Here's how the part is built. I have some questions about the finished solid (model axes, mm). A direction names the side the tool comes from. Coordinates: 2 decimals unless noted, no trailing zeros. Write each loop counter-clockwise with the first axis right and the second up, starting at its lowest first coordinate (ties: lowest second). Pieces come first, ordered by that corner, then holes.
Item 1: If we mould it in two halves opening along X, with no side actions, what happens to faces 1 (the face through (2, 70, 1)), 2 (the face through (-0.2, -44, 2)), 3 (the face through (0, 68, 1)), 4 (the face through (-15, -51, 1))? For each: pulls with the +X half, pulls with the -X half, needs draft (parallel to the pull), parting line crosses it, or undercut.
Item 2: I want a section at C-C (z = 1.75). Count the separate pieces of the cut face and the enclosed holes in it, and give its area (3 significant figures).
Item 3: I'm going to push flat-ended pins straight in: P1, Ø12, axis at x = -1.5, y = -0.5, coming from the -Z side; P2, Ø1.5, axis at y = -43, z = 1, coming from the +X side; P3, Ø1, axis at y = 17, z = 1.5, coming from the +X side; P4, Ø0.9, axis at x = -3.5, z = 1.5, coming from the +Y side. Where does each tip first touch, or does it pass through?
Item 4: Please list where these lines run through material, in increasing order: line 1 (Y direction, x = -1.5, z = 1.25); line 2 (Y direction, x = -10.25, z = 2.85); line 3 (X direction, y = 55.5, z = 1.5).
Item 5: I want a section at A-A (x = -8.75). Please give me the cut outline in (y, z), and give its area (3 significant figures).
Item 6: For faces 5 (the face through (-10, -50, 1)), 6 (the face through (-0.2, 61, 2)), 7 (the face through (-10, 69, 1)), 8 (the face through (-12, -52, 1)), which set-ups out of +Z, -Z, +X, -X, +Y, -Y let a thin tool reach every point of the face, with its end or its side?
Item 7: I want a section at B-B (x = -4). Please give me the cut outline in (y, z), and give its area (3 significant figures).
from build123d import *

# Parameters (mm, degrees)
CROQUIS1_W              = 10
CROQUIS1_H              = 3
SALIENTE_EXTRUIR1_DEPTH = 3
CROQUIS2_W              = 0.3
CROQUIS2_H              = 0.3
CROQUIS2_H_2            = 3
CORTAR_EXTRUIR2_DEPTH   = 3


with BuildPart() as part:
    # Croquis1 → Saliente-Extruir1 (new body)
    with BuildSketch(Plane.XY):
        with BuildLine():
            Line((-10, 70), (-10, 67))
            Line((-10, 67), (-7, 67))
            Line((-7, 67), (-7, 63))
            Line((-7, 63), (-9.5, 63))
            Line((-9.5, 63), (-9.5, 60))
            Line((-9.5, 60), (-0.5, 60))
            Line((-0.5, 60), (-0.5, 63))
            Line((-0.5, 63), (-3, 63))
            Line((-3, 63), (-3, 67))
            Line((-3, 67), (0, 67))
            Line((0, 67), (0, 70))
            Line((0, 70), (5, 70))
            Line((5, 70), (5, 67.405747627))
            ThreePointArc((5, 67.405747627), (4.929306729, 67.036438809), (4.727221995, 66.719345288))
            add(Edge.make_bspline(
                [(4.727221995, 66.719345288), (3.242407332, 65.146230192), (1.757592668, 62), (3.242407332, 58.853769808), (4.727221995, 57.280654712)],
                knots=[0.028065471, 0.028065471, 0.028065471, 0.028065471, 0.5, 0.971934529, 0.971934529, 0.971934529, 0.971934529], degree=3))
            ThreePointArc((4.727221995, 57.280654712), (4.929306729, 56.963561191), (5, 56.594252373))
            Line((5, 56.594252373), (5, 54.181314171))
            ThreePointArc((5, 54.181314171), (4.9841425, 54.003934523), (4.937072921, 53.832180471))
            add(Edge.make_bspline(
                [(4.937072921, 53.832180471), (3.31235764, 49.471453647), (1.68764236, 40.75), (3.31235764, 32.028546353), (4.937072921, 27.667819529)],
                knots=[0.006332812, 0.006332812, 0.006332812, 0.006332812, 0.5, 0.993667188, 0.993667188, 0.993667188, 0.993667188], degree=3))
            ThreePointArc((4.937072921, 27.667819529), (4.9841425, 27.496065477), (5, 27.318685829))
            Line((5, 27.318685829), (5, 24.567654138))
            ThreePointArc((5, 24.567654138), (4.997723384, 24.500214919), (4.990903903, 24.433082766))
            add(Edge.make_bspline(
                [(4.990903903, -48.933082766), (3.330301301, -36.70538851), (1.669698699, -12.25), (3.330301301, 12.20538851), (4.990903903, 24.433082766)],
                knots=[0.000910439, 0.000910439, 0.000910439, 0.000910439, 0.5, 0.999089561, 0.999089561, 0.999089561, 0.999089561], degree=3))
            ThreePointArc((4.990903903, -48.933082766), (4.997723384, -49.000214919), (5, -49.067654138))
            Line((5, -49.067654138), (5, -51.701381229))
            Line((5, -51.701381229), (5, -52))
            Line((5, -52), (0, -52))
            Line((0, -52), (0, -49))
            Line((0, -49), (-3, -49))
            Line((-3, -49), (-3, -45.5))
            Line((-3, -45.5), (-0.5, -45.5))
            Line((-0.5, -45.5), (-0.5, -42.5))
            Line((-0.5, -42.5), (-9.5, -42.5))
            Line((-9.5, -42.5), (-9.5, -45.5))
            Line((-9.5, -45.5), (-7, -45.5))
            Line((-7, -45.5), (-7, -49))
            Line((-7, -49), (-10, -49))
            Line((-10, -49), (-10, -52))
            Line((-10, -52), (-15, -52))
            Line((-15, -52), (-15, -51.701381229))
            Line((-15, -51.701381229), (-15, -49.067654138))
            ThreePointArc((-15, -49.067654138), (-14.997723384, -49.000214919), (-14.990903903, -48.933082766))
            add(Edge.make_bspline(
                [(-14.990903903, -48.933082766), (-13.330301301, -36.70538851), (-11.669698699, -12.25), (-13.330301301, 12.20538851), (-14.990903903, 24.433082766)],
                knots=[0.000910439, 0.000910439, 0.000910439, 0.000910439, 0.5, 0.999089561, 0.999089561, 0.999089561, 0.999089561], degree=3))
            ThreePointArc((-14.990903903, 24.433082766), (-14.997723384, 24.500214919), (-15, 24.567654138))
            Line((-15, 24.567654138), (-15, 27.318685829))
            ThreePointArc((-15, 27.318685829), (-14.9841425, 27.496065477), (-14.937072921, 27.667819529))
            add(Edge.make_bspline(
                [(-14.937072921, 53.832180471), (-13.31235764, 49.471453647), (-11.68764236, 40.75), (-13.31235764, 32.028546353), (-14.937072921, 27.667819529)],
                knots=[0.006332812, 0.006332812, 0.006332812, 0.006332812, 0.5, 0.993667188, 0.993667188, 0.993667188, 0.993667188], degree=3))
            ThreePointArc((-14.937072921, 53.832180471), (-14.9841425, 54.003934523), (-15, 54.181314171))
            Line((-15, 54.181314171), (-15, 56.594252373))
            ThreePointArc((-15, 56.594252373), (-14.929306729, 56.963561191), (-14.727221995, 57.280654712))
            add(Edge.make_bspline(
                [(-14.727221995, 57.280654712), (-13.242407332, 58.853769808), (-11.757592668, 62), (-13.242407332, 65.146230192), (-14.727221995, 66.719345288)],
                knots=[0.028065471, 0.028065471, 0.028065471, 0.028065471, 0.5, 0.971934529, 0.971934529, 0.971934529, 0.971934529], degree=3))
            ThreePointArc((-14.727221995, 66.719345288), (-14.929306729, 67.036438809), (-15, 67.405747627))
            Line((-15, 67.405747627), (-15, 70))
            Line((-15, 70), (-10, 70))
        make_face()
        with Locations((-5, 26)):
            Rectangle(CROQUIS1_W, CROQUIS1_H, mode=Mode.SUBTRACT)
        with Locations((-5, 55.5)):
            Rectangle(CROQUIS1_W, CROQUIS1_H, mode=Mode.SUBTRACT)
    extrude(amount=SALIENTE_EXTRUIR1_DEPTH)

    # Croquis2 → Cortar-Extruir2 (cut)
    with BuildSketch(Plane.XY.offset(3)):
        Polygon((-9.8, -45.5), (-9.8, -45.8), (-9.5, -45.8), (-7, -45.8), (-7, -45.5), (-9.5, -45.5), (-9.5, -42.5), (-0.5, -42.5), (-0.5, -42.2), (-9.5, -42.2), (-9.8, -42.2), (-9.8, -42.5), align=None)
        Polygon((-0.5, -45.8), (-0.2, -45.8), (-0.2, -45.5), (-0.2, -42.5), (-0.5, -42.5), (-0.5, -45.5), (-3, -45.5), (-3, -45.8), align=None)
        with Locations((-0.35, -42.35)):
            Rectangle(CROQUIS2_W, CROQUIS2_H)
        with Locations((-10.15, 26)):
            Rectangle(CROQUIS2_W, CROQUIS2_H_2)
        with Locations((0.15, 26)):
            Rectangle(CROQUIS2_W, CROQUIS2_H_2)
        with Locations((0.15, 55.5)):
            Rectangle(CROQUIS2_W, CROQUIS2_H_2)
        with Locations((-10.15, 55.5)):
            Rectangle(CROQUIS2_W, CROQUIS2_H_2)
        Polygon((-9.8, 63.3), (-9.5, 63.3), (-7, 63.3), (-7, 63), (-9.5, 63), (-9.5, 60), (-0.5, 60), (-0.5, 63), (-3, 63), (-3, 63.3), (-0.5, 63.3), (-0.2, 63.3), (-0.2, 63), (-0.2, 60), (-0.2, 59.7), (-0.5, 59.7), (-9.5, 59.7), (-9.8, 59.7), (-9.8, 60), (-9.8, 63), align=None)
    extrude(amount=-CORTAR_EXTRUIR2_DEPTH, mode=Mode.SUBTRACT)


solid = part.part
Answer:
1. face 1: needs draft
1. face 2: undercut
1. face 3: undercut
1. face 4: pulls with the -X half
2. separate pieces: 1
2. enclosed holes: 2
2. area: 1,850 mm2
3. P1: stops at z = 0
3. P2: stops at x = 4.34
3. P3: stops at x = 4.14
3. P4: stops at y = 59.7
4. line 1: y = -49 to -45.8, -42.2 to 24.5, 27.5 to 54, 57 to 59.7, 63.3 to 67
4. line 2: y = -52 to 24.5, 27.5 to 54, 57 to 70
4. line 3: x = -15 to -10.3, 0.3 to 5
5. outline: (-49, 0) - (-45.8, 0) - (-45.8, 3) - (-49, 3) - close; (-42.2, 0) - (24.5, 0) - (24.5, 3) - (-42.2, 3) - close; (27.5, 0) - (54, 0) - (54, 3) - (27.5, 3) - close; (57, 0) - (59.7, 0) - (59.7, 3) - (57, 3) - close; (63.3, 0) - (67, 0) - (67, 3) - (63.3, 3) - close
5. area: 308 mm2
6. face 5: +Z, -Z, -Y
6. face 6: +Z, -Z
6. face 7: +Z, -Z, +Y
6. face 8: +Z, -Z, +X, -X, -Y
7. outline: (-42.2, 0) - (24.5, 0) - (24.5, 3) - (-42.2, 3) - close; (27.5, 0) - (54, 0) - (54, 3) - (27.5, 3) - close; (57, 0) - (59.7, 0) - (59.7, 3) - (57, 3) - close
7. area: 288 mm2
